Geometry: see drawing. Coordinates: mm, zero at the bounding-box minimum. Round coordinates to 2 decimals unless told otherwise and drop trailing zeros. Order: outer loops, then holes, each group sorted by start corner. A loop starts at its lowest first (then second) coordinate and runs counter-clockwise, first axis right, second up. Notation, with made-up numbers: (47, -38) -> (61, -38) arc R7 cw to (61, -30) -> close; hole circle Ø6 at (-24, -19). An arc over 180 degrees is marked (long way). Answer as CSV lines item,"result". Start each with the question number.
(1) Section query D-D (y = 15). Output: boundary loops of the cut face in (x, z), plus the area to 3 significant figures.
(2) Contact query for flat-ended pins moving along their axis: P1, Ø4, axis at x = 5, y = 5, coming from the -Z side; P2, Ø1.5, axis at y = 5, z = 2, coming from the +X side; P3, Ø1.5, axis at y = 5.5, z = 2.5, coming from the +X side. Output: stop coordinate, or through.
(3) Pull-direction query (X, two-part tool) for the marked faces 1, 2 and 3; classes: +X half, -X half, draft (parallel to the pull), parting line (faces both ways), or undercut.
(4) Section query C-C (z = 1.8). Output: boundary loops of the cut face in (x, y).
(5) Section query A-A (y = 10). Output: boundary loops of the cut face in (x, z), plus the area to 3 significant figures.
(6) Line query: line 1 along Y through (x, z) = (10, 2.05); line 2 along X through (y, z) = (5.5, 1.2); line 3 along Y through (x, z) = (16, 1.15). Output: solid intervals per line, ascending. Write a range as from..to.
(7) Section query B-B (x = 10.75). Output: boundary loops of the cut face in (y, z), plus the area to 3 significant figures.
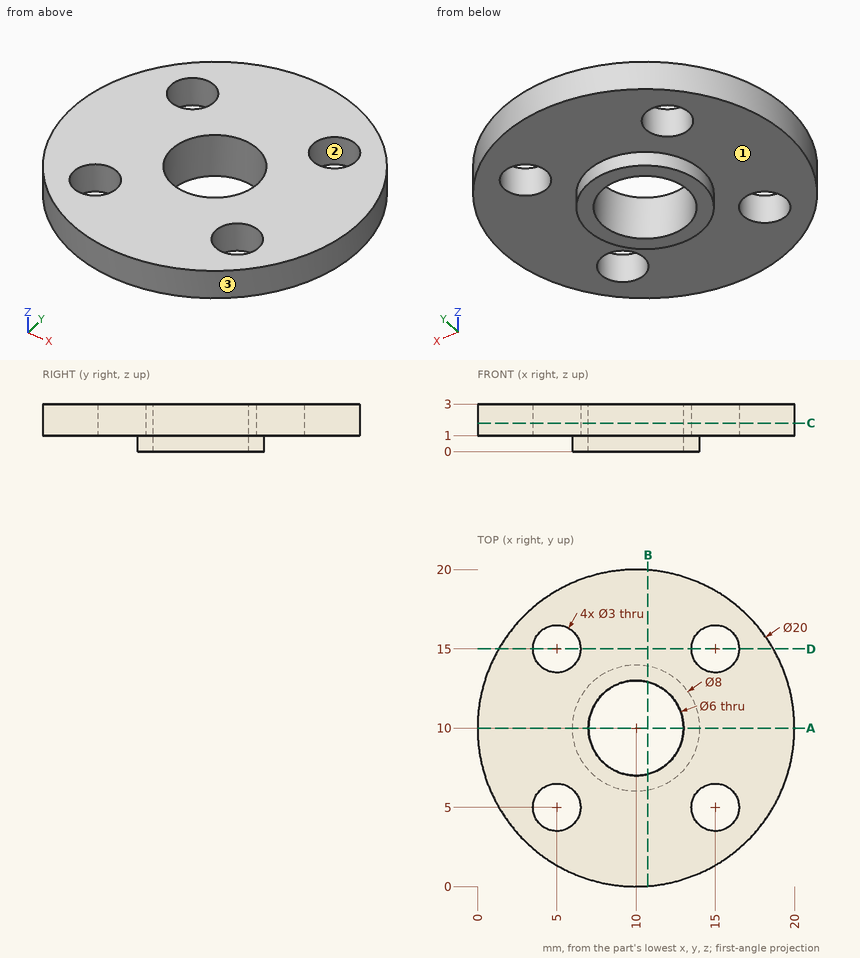
Answer block:
1,outline,"(1.34, 1) -> (3.5, 1) -> (3.5, 3) -> (1.34, 3) -> close; (6.5, 1) -> (13.5, 1) -> (13.5, 3) -> (6.5, 3) -> close; (16.5, 1) -> (18.66, 1) -> (18.66, 3) -> (16.5, 3) -> close"
1,area,"22.6 mm2"
2,P1,"z = 1"
2,P2,"x = 19.05"
2,P3,"x = 19.27"
3,face 1,"draft"
3,face 2,"undercut"
3,face 3,"parting line"
4,outline,"circle Ø20 at (10, 10); hole circle Ø3 at (5, 5); hole circle Ø3 at (5, 15); hole circle Ø6 at (10, 10); hole circle Ø3 at (15, 5); hole circle Ø3 at (15, 15)"
5,outline,"(0, 1) -> (6, 1) -> (6, 0) -> (7, 0) -> (7, 3) -> (0, 3) -> close; (13, 0) -> (14, 0) -> (14, 1) -> (20, 1) -> (20, 3) -> (13, 3) -> close"
5,area,"30.0 mm2"
6,line 1,"0..7, 13..20"
6,line 2,"1.07..3.59, 6.41..13.59, 16.41..18.93"
6,line 3,"2..3.88, 6.12..13.88, 16.12..18"
7,outline,"(0.03, 1) -> (6.07, 1) -> (6.07, 0) -> (7.1, 0) -> (7.1, 3) -> (0.03, 3) -> close; (12.9, 0) -> (13.93, 0) -> (13.93, 1) -> (19.97, 1) -> (19.97, 3) -> (12.9, 3) -> close"
7,area,"30.3 mm2"
